Autodesk Inventor part; units mm, degrees
ref_plane "YZ Plane" through (0, 0, 0) normal (1, 0, 0) x (0, 1, 0)
ref_plane "XZ Plane" through (0, 0, 0) normal (0, 1, 0) x (-1, 0, 0)
ref_plane "XY Plane" through (0, 0, 0) normal (0, 0, 1) x (1, 0, 0)
sketch "Szkic1" plane through (0, 0, 0) normal (0, 0, 1) x (1, 0, 0)
  line L0 (0, 0) -> (20, 0)
  line L1 (20, 0) -> (20, 40)
  line L2 (20, 40) -> (0, 40)
  line L3 (0, 40) -> (0, 0)
  circle A0 centre (10, 20) radius 3
  dimension "d0" = 20
  dimension "d1" = 40
  dimension "d2" = 6
extrude "Wyciągnięcie proste1" add sketch "Szkic1" along normal blind 49
sketch "Szkic2" plane through (0, 0, 49) normal (0, 0, 1) x (1, 0, 0)
  line L0 (3, 37) -> (17, 37)
  line L1 (17, 37) -> (17, 3)
  line L2 (17, 3) -> (3, 3)
  line L3 (3, 3) -> (3, 37)
  line L4 (0, 0) -> (20, 0)
  line L5 (20, 40) -> (0, 40)
  line L6 (0, 40) -> (0, 0)
  line L7 (20, 0) -> (20, 40)
  dimension "d5" = 14
  dimension "d6" = 34
  dimension "d7" = 3
  dimension "d8" = 3
  dimension "d9" = 3
  dimension "d10" = 3
extrude "Wyciągnięcie proste2" cut sketch "Szkic2" against normal blind 46 contours L0 L1 L2 L3
sketch "Szkic3" plane through (0, 0, 49) normal (0, 0, 1) x (1, 0, 0)
  line L0 (3, 3) -> (3, 37)
  line L1 (3, 37) -> (17, 37)
  line L2 (3, 3) -> (17, 3)
  line L3 (17, 3) -> (17, 37)
  line L4 (17, 37) -> (3, 37)
  line L5 (3, 37) -> (3, 3)
  line L6 (17, 3) -> (3, 3) construction
  line L7 (3, 3) -> (3, 1.5) construction
  line L8 (3, 1.5) -> (1.5, 1.5) construction
  line L9 (1.5, 1.5) -> (18.5, 1.5)
  line L10 (18.5, 1.5) -> (18.5, 38.5)
  line L11 (18.5, 38.5) -> (1.5, 38.5)
  line L12 (1.5, 38.5) -> (1.5, 1.5)
  point P0 (0, 0)
  dimension "d13" = 1.5
  dimension "d14" = 1.5
  dimension "d15" = 34
  dimension "d16" = 14
  dimension "d17" = 17
  dimension "d18" = 37
extrude "Wyciągnięcie proste3" add sketch "Szkic3" along normal blind 10
sketch "Szkic4" plane through (0, 0, 0) normal (-1, 0, 0) x (0, 0, 1)
  line L0 (0, 0) -> (0, 20)
  line L1 (0, 0) -> (0, 40)
  line L2 (0, 20) -> (16.8, 20)
  circle A0 centre (16.8, 20) radius 10
  dimension "d21" = 16.8
  dimension "d22" = 20
extrude "Wyciągnięcie proste4" cut sketch "Szkic4" against normal up to surface (3 mm away)
sketch "Szkic5" plane through (1.5, 1.5, 49) normal (-1, 0, 0) x (0, 0, 1)
  line L0 (0, 0) -> (10, 0) construction
  line L1 (0, 37) -> (10, 37) construction
  line L2 (10, 0) -> (0, 37) construction
  line L3 (0, 37) -> (10, 37) construction
  line L4 (10, 37) -> (0, 0) construction
  line L5 (0, 38.5) -> (0, -1.5) construction
  line L6 (5.5, 20.5) -> (4.5, 20.5)
  line L7 (4.5, 20.5) -> (4.5, 16.5)
  line L8 (4.5, 16.5) -> (5.5, 16.5)
  line L9 (5.5, 16.5) -> (5.5, 20.5)
  line L10 (5.5, 20.5) -> (4.5, 16.5) construction
  line L11 (4.5, 20.5) -> (5.5, 16.5) construction
  point P0 (-49, -1.5)
  point P1 (5, 18.5)
  dimension "d25" = 1
  dimension "d26" = 4
  dimension "d29" = 4.5
extrude "Wyciągnięcie proste5" cut sketch "Szkic5" against normal up to surface (1.5 mm away)
equation "\"d7\" = d8"
equation "\"d9\" = d10"
equation "\"d14\" = d13"
equation "\"d17\" = d16 + 2 * d14"
equation "\"d18\" = d15 + 2 * d14"
properties part number "obudowa_latarka"
Work out the finished part from the listing and answer in its coordinate system (mm). A direction names the side the tool comes from. Round coordinates to 2 decimals unless told otherwise and drop trailing zeros. Write each loop counter-clockwise with the first axis right and the second up, starting at its lowest first coordinate (ties: lowest second). Pieces come first, ordered by that corner, then holes. Notation, with made-up numbers: (-6, 33) - (13, 33) arc R24 ccw to (13, 56) - close; hole circle Ø5 at (50, -6.5). An arc over 180 degrees is marked (long way). Return JSON: item names as keys, results as strings. Group by question number.
Q1. Each of these flat-tipped pins is pushed along its axis until it touches: pin 1 Ø0.8 at (x, z) = (2, 54) entering from +Y; pin 2 Ø11 at (y, z) = (26, 56) entering from +X; pin 3 Ø5 at (x, z) = (11.5, 55) entering from -Y. Where does it stop, or does it pass through?
Q2. The part is cut by section D-D on y = 20. Write down the section's boundary in (x, z).
Q3. The part is cut by section C-C on y = 15.5. Write down the section's boundary in (x, z).
Q4. Find the intervals of material crossed by L1, parallel to Y at x = 6, z = 25.5; L2, parallel to Z at x = 1.6, y = 20; L3, parallel to Y at x = 10, z = 1, in increasing order.
Q5. For faces 1 (the flat face through (10, 37, 31)), 2 (the flat face through (1.5, 20, 53)), 3 (the flat face through (2, 20, 54.5)), determine the directions among +Z, -Z, +X, -X, +Y, -Y from which every point of the face is accessible in a straight line to the end or side of a thin tool.
Q6. The part is cut by section A-A on x = 10. Write down the section's boundary in (y, z).
Q7. The mould has two halves that part along Z. Classify faces 4 (the cylindrical face through (1.479, 29.915, 15.498)), 5 (the flat face through (6.8, 20.2, 3)), 6 (the flat face through (17, 20, 31)), 7 (the flat face through (2, 20, 53.5)): released by +Z, released by -Z, zero draft, split by the parting line, or undercut.
Q8. The part is cut by section B-B on z = 37.5. Write down the section's boundary in (x, y), then the cut area to 3 significant figures.
Solved:
{
 "1": {"pin 1": "y = 38.5", "pin 2": "x = 18.5", "pin 3": "y = 1.5"},
 "2": {"outline": "(0, 0) - (7, 0) - (7, 3) - (3, 3) - (3, 6.8) - (0, 6.8) - close; (0, 26.8) - (3, 26.8) - (3, 53.5) - (1.5, 53.5) - (1.5, 49) - (0, 49) - close; (1.5, 54.5) - (3, 54.5) - (3, 59) - (1.5, 59) - close; (13, 0) - (20, 0) - (20, 49) - (18.5, 49) - (18.5, 59) - (17, 59) - (17, 3) - (13, 3) - close"},
 "3": {"outline": "(0, 0) - (20, 0) - (20, 49) - (18.5, 49) - (18.5, 59) - (17, 59) - (17, 3) - (3, 3) - (3, 7.87) - (0, 7.87) - close; (0, 25.73) - (3, 25.73) - (3, 59) - (1.5, 59) - (1.5, 49) - (0, 49) - close"},
 "4": {"L1": "0 to 3, 37 to 40", "L2": "0 to 6.8, 26.8 to 53.5, 54.5 to 59", "L3": "0 to 17, 23 to 40"},
 "5": {"face 1": "+Z", "face 2": "+Z, -X, +Y, -Y", "face 3": "-X"},
 "6": {"outline": "(0, 0) - (17, 0) - (17, 3) - (3, 3) - (3, 59) - (1.5, 59) - (1.5, 49) - (0, 49) - close; (23, 0) - (40, 0) - (40, 49) - (38.5, 49) - (38.5, 59) - (37, 59) - (37, 3) - (23, 3) - close"},
 "7": {"face 4": "undercut", "face 5": "released by +Z", "face 6": "zero draft", "face 7": "undercut"},
 "8": {"outline": "(0, 0) - (20, 0) - (20, 40) - (0, 40) - close; hole (3, 3) - (17, 3) - (17, 37) - (3, 37) - close", "area": "324 mm²"}
}
